```python
from build123d import *

# Parameters (mm, degrees)
SKETCH1_W           = 54.74
SKETCH1_H           = 81.28
SKETCH1_R           = 1.7
SKETCH1_R_2         = 0.83
BOSS_EXTRUDE1_DEPTH = 1.5
SKETCH2_W           = 51.5
SKETCH2_H           = 70.7
BOSS_EXTRUDE2_DEPTH = 2.9
BOSS_EXTRUDE3_DEPTH = 2.54


with BuildPart() as part:
    # Sketch1 → Boss-Extrude1 (new body)
    with BuildSketch(Plane(origin=(0, 0, 0), x_dir=(1, 0, 0), z_dir=(0, 1, 0))):
        Rectangle(SKETCH1_W, SKETCH1_H)
        with Locations(Location((-25.01, 38.28, 0), (0, 0, 270))):
            Circle(SKETCH1_R, mode=Mode.SUBTRACT)
        with Locations(Location((25.01, 38.28, 0), (0, 0, 90))):
            Circle(SKETCH1_R, mode=Mode.SUBTRACT)
        with Locations(Location((-25.01, -38.28, 0), (0, 0, 90))):
            Circle(SKETCH1_R, mode=Mode.SUBTRACT)
        with Locations(Location((25.01, -38.28, 0), (0, 0, 270))):
            Circle(SKETCH1_R, mode=Mode.SUBTRACT)
        with Locations(Location((0, 38.28, 0), (0, 0, 270))):
            Circle(SKETCH1_R_2, mode=Mode.SUBTRACT)
        with Locations(Location((2.54, 38.28, 0), (0, 0, 270))):
            Circle(SKETCH1_R_2, mode=Mode.SUBTRACT)
        with Locations(Location((5.08, 38.28, 0), (0, 0, 270))):
            Circle(SKETCH1_R_2, mode=Mode.SUBTRACT)
        with Locations(Location((7.62, 38.28, 0), (0, 0, 270))):
            Circle(SKETCH1_R_2, mode=Mode.SUBTRACT)
        with Locations(Location((-2.54, 38.28, 0), (0, 0, 270))):
            Circle(SKETCH1_R_2, mode=Mode.SUBTRACT)
        with Locations(Location((-5.08, 38.28, 0), (0, 0, 270))):
            Circle(SKETCH1_R_2, mode=Mode.SUBTRACT)
        with Locations(Location((-7.62, 38.28, 0), (0, 0, 270))):
            Circle(SKETCH1_R_2, mode=Mode.SUBTRACT)
    extrude(amount=BOSS_EXTRUDE1_DEPTH)

    # Sketch2 → Boss-Extrude2 (add)
    with BuildSketch(Plane(origin=(0, 1.5, 0), x_dir=(1, 0, 0), z_dir=(0, 1, 0))):
        Rectangle(SKETCH2_W, SKETCH2_H)
    extrude(amount=BOSS_EXTRUDE2_DEPTH)

    # Sketch3 → Boss-Extrude3 (add)
    with BuildSketch(Plane.XZ):
        Polygon((-6.35, -37.01), (6.35, -37.01), (8.89, -37.01), (8.89, -39.55), (6.35, -39.55), (-6.35, -39.55), (-8.89, -39.55), (-8.89, -37.01), align=None)
    extrude(amount=BOSS_EXTRUDE3_DEPTH)


solid = part.part
```
Input: part model. Units: mm. Frame: model coordinates. A direction names the side the tool comes from. Give positions to 0.01 mm unless a question says otherwise; leave off trailing zeros. Loops run counter-clockwise (first coordinate to the right, second up) from the corner with the lowest first, then second, coordinate; pieces in that order, holes last.
1) Mould query, pull axis X, two halves, no side actions, for faces 1 (the cylindrical face through (0.823, 0.74, -38.388)), 2 (the flat face through (27.37, 1, 1)), 3 (the cylindrical face through (6.81, 0.74, -38.46)), 4 (the flat face through (0, -2.54, -38)). Classes: released by +X, released by -X, zero draft, split by the parting line, or undercut.
A:
face 1: undercut
face 2: released by +X
face 3: undercut
face 4: zero draft
2) Section query C-C on y = -1. Return the cut outline in (x, z).
A:
outline: (-8.89, -39.55) - (8.89, -39.55) - (8.89, -37.01) - (-8.89, -37.01) - close
3) Section query B-B on x = 18.5. Return the cut outline in (y, z).
A:
outline: (0, -40.64) - (1.5, -40.64) - (1.5, -35.35) - (4.4, -35.35) - (4.4, 35.35) - (1.5, 35.35) - (1.5, 40.64) - (0, 40.64) - close
4) Section query D-D on z = -38.28. Count the separate pieces of the cut face and the enclosed holes in it, and give its area (3 significant figures).
A:
separate pieces: 3
enclosed holes: 0
area: 99.6 mm2
5) Section query A-A on z = 38.28. Return the cut outline in (x, y).
A:
outline: (-27.37, 0) - (-26.71, 0) - (-26.71, 1.5) - (-27.37, 1.5) - close; (-23.31, 0) - (23.31, 0) - (23.31, 1.5) - (-23.31, 1.5) - close; (26.71, 0) - (27.37, 0) - (27.37, 1.5) - (26.71, 1.5) - close
6) Line query: L1, parallel to Y at x = -10.5, z = 17.5; L2, parallel to Z at x = 19, y = 2; L3, parallel to X at y = 2.25, z = 5. Output: solid intervals per line, ascending.
A:
L1: y = 0 to 4.4
L2: z = -35.35 to 35.35
L3: x = -25.75 to 25.75
7) Reachability of faces 5 (the flat face through (25.75, 3, 0)), 6 (the flat face through (-8.89, -1, -38)), 7 (the flat face through (5, 0, -38)), 8 (the flat face through (0, -1, -39.55)) from +Z, -Z, +X, -X, +Y, -Y: full face, straight path, thin tool, end or side. Return the list, or none.
A:
face 5: +Z, -Z, +X, +Y
face 6: +Z, -Z, -X, -Y
face 7: +Y
face 8: -Z, +X, -X, -Y
8) Contact query for flat-ended pins moving along their axis: pin 1 (1.8 mm diameter, centred on x = 5.5, z = -38, fed in from +Y); pin 2 (1.3 mm diameter, centred on y = -1, z = -38.5, fed in from +X); pin 3 (4 mm diameter, centred on y = -1, z = -21, fed in from -X); pin 4 (0.5 mm diameter, centred on x = 0, z = -38, fed in from +Y). Output: stop coordinate, or through.
A:
pin 1: stops at y = 1.5
pin 2: stops at x = 8.89
pin 3: stops at x = -27.37
pin 4: stops at y = 0
